The model under review builds one solid part; all positions refer to its coordinate system, in mm. A direction names the side the tool comes from. Round coordinates to 2 decimals unless told otherwise and drop trailing zeros. Write each loop counter-clockwise with the first axis right and the second up, starting at its lowest first coordinate (ties: lowest second). Pieces come first, ordered by that corner, then holes. Notation, with made-up numbers: (87.5, 81) - (140.5, 81) arc R31 ccw to (140.5, 113) - close; hole circle Ø10 at (83, -32). An arc over 180 degrees is marked (long way). Use one line per item in the form item = value.
from build123d import *

# Parameters (mm, degrees)
BOSS_EXTRUDE1_DEPTH = 2
CIRPATTERN1_COUNT   = 8


with BuildPart() as part:
    # Sketch1 → Boss-Extrude1 (new body)
    with BuildSketch(Plane(origin=(0, 0, 0), x_dir=(1, 0, 0), z_dir=(0, 1, 0))):
        with BuildLine():
            Line((28.994949366, -70), (70, -28.994949366))
            Line((70, -28.994949366), (70, 28.994949366))
            Line((70, 28.994949366), (28.994949366, 70))
            Line((28.994949366, 70), (1.798096452, 70))
            ThreePointArc((1.798096452, 70), (-15.601802765, 75.561434018), (-26.550475887, 90.183766184))
            ThreePointArc((-26.550475887, 90.183766184), (-39.826834324, 96.150483571), (-44.995531078, 82.543574165))
            ThreePointArc((-44.995531078, 82.543574165), (-42.397861857, 64.462142924), (-50.768920878, 48.226028488))
            Line((-50.768920878, 48.226028488), (-70, 28.994949366))
            Line((-70, 28.994949366), (-70, -28.994949366))
            Line((-70, -28.994949366), (-28.994949366, -70))
            Line((-28.994949366, -70), (28.994949366, -70))
        make_face()
    boss_extrude1 = extrude(amount=BOSS_EXTRUDE1_DEPTH)

    # CirPattern1: Boss-Extrude1 ×8 about axis
    cirpattern1_axis = Axis((0, 0, 0), (0, 1, 0))
    for i in range(1, CIRPATTERN1_COUNT):
        add(boss_extrude1.rotate(cirpattern1_axis, i * 360 / CIRPATTERN1_COUNT))


solid = part.part
(1) Add section D-D on z = -55. Write out the cut boundary in (x, y).
Geometry results:
outline = (-45.69, 0) - (45.69, 0) - (45.69, 2) - (-45.69, 2) - close
(2) Machinability: for faces 4 (the cylindrical face through (-16.129, 0.986, -75.946)), 5 (the cylindrical face through (76.24, 0.99, 16.52)), 6 (the flat face through (0, 2, -2)), which of the approach directions +Z, -Z, +X, -X, +Y, -Y give a long, thin tool a straight path to every point of the face, cutting with its end or side? Answer none if there is none.
Geometry results:
face_4 = -Z, +Y, -Y
face_5 = +X, +Y, -Y
face_6 = +Z, -Z, +X, -X, +Y
(3) The part is to be moulded in two halves that separate along X. For faces 1 (the cylindrical face through (42.297, 0.986, -65.107)), 2 (the cylindrical face through (-75.946, 0.986, 16.129)), 3 (the cylindrical face through (16.129, 0.986, 75.946)), say which applies: +X half, -X half, draft (parallel to the pull), parting line (faces both ways), or undercut.
Geometry results:
face_1 = +X half
face_2 = -X half
face_3 = undercut
(4) Add section C-C on x = 21.5. Write out the cut boundary in (y, z).
Geometry results:
outline = (0, -81.1) - (2, -81.1) - (2, 81.1) - (0, 81.1) - close
(5) To check wall thickness, follow L1, parallel to Z at x = 79, y = 0.55; L2, parallel to Z at x = 37, y = 0.95; L3, parallel to X at y = 1.35, z = -73. State the ranges of each line that lie inside material, in increasing order.
Geometry results:
L1 = -43.55 to -19.63, 19.63 to 43.55
L2 = -96.86 to 96.86
L3 = -42.19 to -11.28, 11.28 to 42.19
(6) Add section A-A on z = 76.5. Write out the cut boundary in (x, y), then the cut area to 3 significant figures.
Geometry results:
outline = (-42.82, 0) - (-16.85, 0) - (-16.85, 2) - (-42.82, 2) - close; (16.85, 0) - (42.82, 0) - (42.82, 2) - (16.85, 2) - close
area = 104 mm2
(7) Add section B-B on y = 1.15. Write out the cut boundary in (x, z), then the cut area to 3 significant figures.
Geometry results:
outline = (-90.18, -26.55) arc R10 ccw (long way) to (-82.54, -45) arc R30 cw to (-49.54, -49.54) arc R30 cw to (-45, -82.54) arc R10 ccw (long way) to (-26.55, -90.18) arc R30 cw to (0, -70.05) arc R30 cw to (26.55, -90.18) arc R10 ccw (long way) to (45, -82.54) arc R30 cw to (49.54, -49.54) arc R30 cw to (82.54, -45) arc R10 ccw (long way) to (90.18, -26.55) arc R30 cw to (70.05, 0) arc R30 cw to (90.18, 26.55) arc R10 ccw (long way) to (82.54, 45) arc R30 cw to (49.54, 49.54) arc R30 cw to (45, 82.54) arc R10 ccw (long way) to (26.55, 90.18) arc R30 cw to (0, 70.05) arc R30 cw to (-26.55, 90.18) arc R10 ccw (long way) to (-45, 82.54) arc R30 cw to (-49.54, 49.54) arc R30 cw to (-82.54, 45) arc R10 ccw (long way) to (-90.18, 26.55) arc R30 cw to (-70.05, 0) arc R30 cw to start
area = 21,900 mm2
(8) Insertion check: P1, Ø1.5, axis at x = 32, z = -28.5, coming from the -Y side. The pin has a flat end and moves straight along its axis. Give the tip position at first contact, or say it passes through.
Geometry results:
P1 = 0
